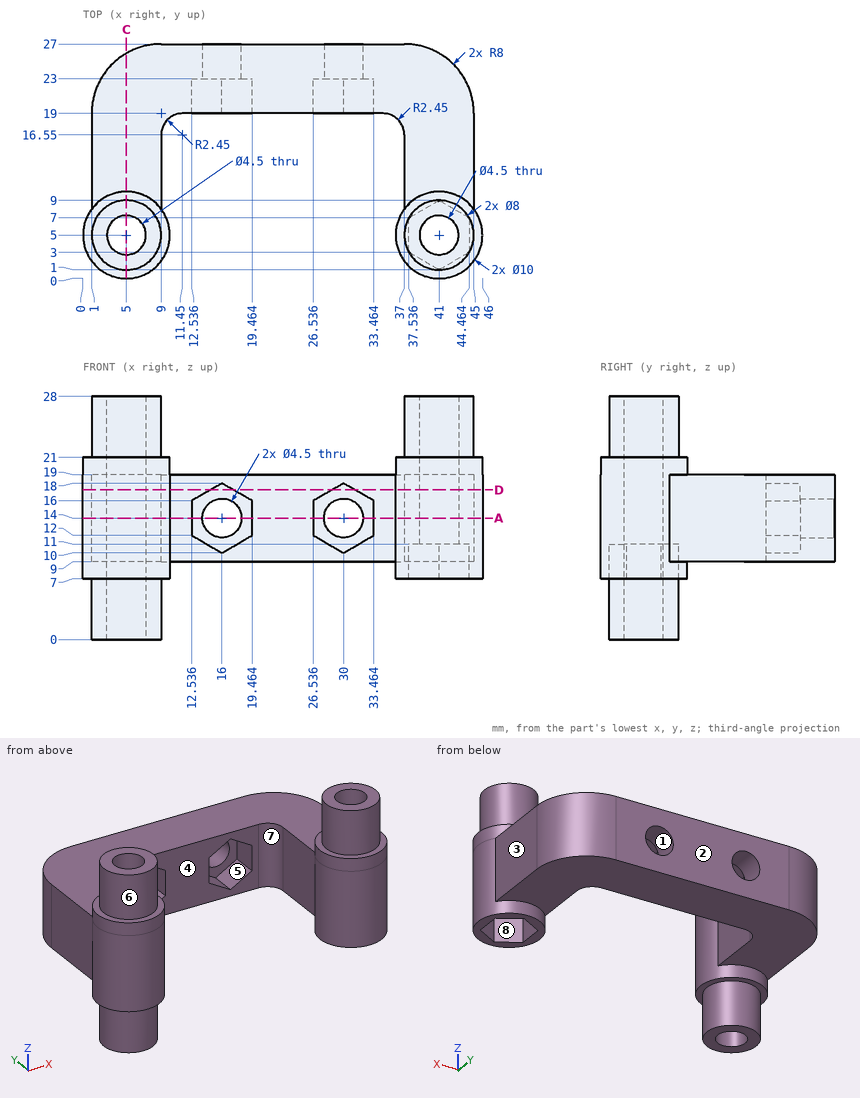
Geometry: see drawing. Coordinates: mm, zero at the bounding-box minimum. A direction names the side the tool comes from. Coordinates: 2 decimals unless noted, no trailing zeros. Loops run counter-clockwise (first coordinate to the right, second up) from the corner with the lowest first, then second, coordinate; pieces in that order, holes last. Notation, with made-up numbers: (25.5, -21.75) - (41.5, -21.75) arc R14 ccw to (41.5, -2.75) - close; hole circle Ø2 at (45, 49). An arc over 180 degrees is marked (long way). Answer as CSV lines item,"result".
1. Mould query, pull axis X, two halves, no side actions, for the marked faces 1, 2 and 3. Classes: released by +X, released by -X, zero draft, split by the parting line, or undercut.
Established:
face 1,"undercut"
face 2,"zero draft"
face 3,"released by +X"
2. Contact query for flat-ended pins moving along their axis: pin 1 (15 mm diameter, centred on x = 24, y = 18, fed in from +Z); pin 2 (4.5 mm diameter, centred on y = 20.5, z = 13.5, fed in from +X); pin 3 (6 mm diameter, centred on y = 11.5, z = 23.5, fed in from -X). Output: stop coordinate, or through.
Established:
pin 1,"stops at z = 19"
pin 2,"stops at x = 45"
pin 3,"stops at x = 3.06"
3. Section C-C (x = 5). Return loops of the section in (y, z), then the cut area to 3 significant figures.
Established:
outline,"(0, 7) - (1, 7) - (1, 0) - (2.75, 0) - (2.75, 28) - (1, 28) - (1, 21) - (0, 21) - close; (7.25, 0) - (9, 0) - (9, 7) - (10, 7) - (10, 9) - (25.93, 9) - (25.93, 19) - (10, 19) - (10, 21) - (9, 21) - (9, 28) - (7.25, 28) - close"
area,"285 mm2"
4. Section D-D (z = 17.25). Return loops of the section in (x, y), then the cut area to 3 significant figures.
Established:
outline,"(1, 8) arc R5 ccw (long way) to (9, 8) - (9, 16.55) arc R2.45 cw to (11.45, 19) - (14.7, 19) - (14.7, 23) - (17.3, 23) - (17.3, 19) - (28.7, 19) - (28.7, 23) - (31.3, 23) - (31.3, 19) - (34.55, 19) arc R2.45 cw to (37, 16.55) - (37, 8) arc R5 ccw (long way) to (45, 8) - (45, 19) arc R8 ccw to (37, 27) - (9, 27) arc R8 ccw to (1, 19) - close; hole circle Ø4.5 at (5, 5); hole circle Ø4.5 at (41, 5)"
area,"585 mm2"
5. Reachability of the marked faces 4, 5, 6, 7 and 8 from +Z, -Z, +X, -X, +Y, -Y: full face, straight path, thin tool, end or side. Return the list, or none.
Established:
face 4,"+Z, -Z, -Y"
face 5,"-Y"
face 6,"+Z"
face 7,"+Z, -Z"
face 8,"-Z"
6. Ray query, line 1 (X direction, y = 5, z = 15.25); line 2 (Y direction, x = 27.5, z = 16.75); line 3 (Z direction, x = 31.5, y = 21.75). Return the intervals inside material, ascending.
Established:
line 1,"x = 0 to 2.75, 7.25 to 10, 36 to 38.75, 43.25 to 46"
line 2,"y = 19 to 27"
line 3,"z = 9 to 10.87, 17.13 to 19"
7. Section A-A (z = 14). Count the separate pieces of the cut face and the enclosed holes in it, then the cut area to 3 significant figures.
Established:
separate pieces,"3"
enclosed holes,"2"
area,"515 mm2"
